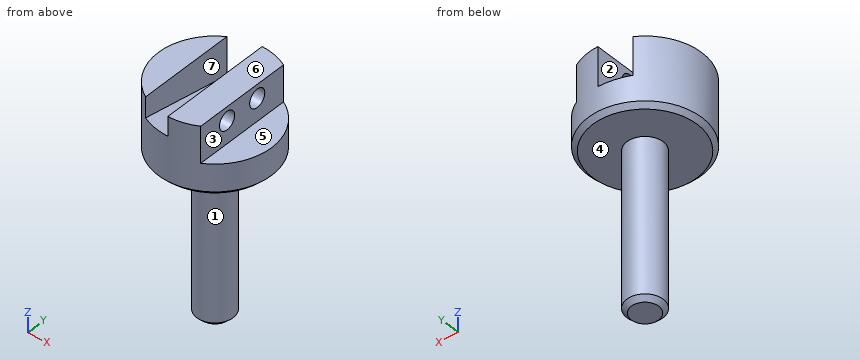
from build123d import *

# Parameters (mm, degrees)
F0_R      = 4
F1_DEPTH  = 35
F2_R      = 12.5
F2_R_2    = 4
F3_DEPTH  = 15
F4_W      = 6.5
F4_H      = 21.9317121995
F5_DEPTH  = 8
F9_W      = 6.35
F9_H      = 60
F10_DEPTH = 25
F11_R     = 2
F12_DEPTH = 8
F13_SIZE  = 1


with BuildPart() as f1:
    # F0 (on Top) → F1 (new body)
    with BuildSketch(Plane.XY):
        Circle(F0_R)
    extrude(amount=F1_DEPTH)

    # F2 (on face) → F3 (join)
    with BuildSketch(Plane.XY.offset(35)):
        Circle(F2_R)
        Circle(F2_R_2, mode=Mode.SUBTRACT)
        Circle(F2_R)
    extrude(amount=F3_DEPTH)

    # F4 (on face) → F5 (cut)
    with BuildSketch(Plane.XY.offset(50)):
        with Locations((9.25, 0)):
            Rectangle(F4_W, F4_H)
    extrude(amount=-F5_DEPTH, mode=Mode.SUBTRACT)

    # F9 (on offset) → F10 (cut)
    with BuildSketch(Plane(origin=(0, 7.447837655, 42.238786288), x_dir=(1, 0, 0), z_dir=(0, 0.1736481777, 0.984807753))):
        with Locations((-3.175, -7.9551495101)):
            Rectangle(F9_W, F9_H)
    extrude(amount=F10_DEPTH, mode=Mode.SUBTRACT)

    # F11 (on face) → F12 (cut)
    with BuildSketch(Plane.YZ.offset(6)):
        with Locations((4, 47)):
            Circle(F11_R)
        with Locations((-4, 47)):
            Circle(F11_R)
    extrude(amount=-F12_DEPTH, mode=Mode.SUBTRACT)

    # F13
    f13_edges = [f1.edges().sort_by_distance(p)[0] for p in [
        (-12.5, 0, 35),
        (-4, 0, 0),
    ]]
    chamfer(f13_edges, length=F13_SIZE)


solid = f1.part
Input: part model. Units: mm. Frame: model coordinates. Face numbers are marked on the shaded views. A direction names the side the tool comes from. Round coordinates to 2 decimals unless told otherwise and drop trailing zeros. Order: outer loops, then holes, each group sorted by start corner. A loop starts at its lowest first (then second) coordinate and runs counter-clockwise, first axis right, second up.
1. Cut plane A-A, the plane z = 47. Output: boundary loops of the cut face in (x, y).
The answers:
outline: (-6.35, -10.77) - (-6.35, 10.77) arc R12.5 ccw to start; (0, -12.5) arc R12.5 ccw to (6, -10.97) - (6, -6) - (0, -6) - close; (0, -2) - (6, -2) - (6, 2) - (0, 2) - close; (0, 6) - (6, 6) - (6, 10.97) arc R12.5 ccw to (0, 12.5) - close
2. Pin query (flat end, axial travel): P1, Ø3.5, axis at x = 9, y = -2.5, coming from the +Z side; P2, Ø1.5, axis at x = -3, y = 7.5, coming from the +Z side; P3, Ø10, axis at x = -3.5, z = 24, coming from the -Y side. Return the tip coordinate at first contact, or that it passes through.
The answers:
P1: stops at z = 42
P2: stops at z = 42.36
P3: stops at y = -4
3. Cut plane C-C, the plane x = 0.75. State how many separate pieces and enclosed holes the cut face has, then the cut area to 3 significant figures.
The answers:
separate pieces: 1
enclosed holes: 2
area: 622 mm2
4. Cut plane B-B, the plane z = 18. Output: boundary loops of the cut face in (x, y), then the cut area to 3 significant figures.
The answers:
outline: circle Ø8 at (0, 0)
area: 50.3 mm2
5. Mould query, pull axis X, two halves, no side actions, for the marked faces 1, 2, 3 and 4. Classes: released by +X, released by -X, zero draft, split by the parting line, or undercut.
The answers:
face 1: split by the parting line
face 2: undercut
face 3: released by +X
face 4: zero draft
6. Set-up query: the marked faces 5, 6 and 7. Return all of +Z, -Z, +X, -X, +Y, -Y with unobstructed straight access to the full face (end or side cutting, diameter ignored); none if empty.
The answers:
face 5: +Z, +X, +Y, -Y
face 6: +Z, +X, -X, +Y, -Y
face 7: +Z, +Y
7. Material intervals for line 1 (Z direction, x = 3.2, y = 4); line 2 (X direction, y = 0.25, z = 26); line 3 (Z direction, x = 4.5, y = -3.25), sorted ascending.
The answers:
line 1: z = 35 to 45, 49 to 50
line 2: x = -3.99 to 3.99
line 3: z = 35 to 45.15, 48.85 to 50
